from build123d import *
from OCP.BRepFilletAPI import BRepFilletAPI_MakeChamfer

# Parameters (mm, degrees)
BOSS_EXTRUDE2_DEPTH           = 26
SKETCH5_R                     = 11
CUT_EXTRUDE1_DEPTH            = 52.857979135
CSK_FOR_M3_SFHCS1_D           = 3.4
CSK_FOR_M3_SFHCS1_CSINK_D     = 6.72
CSK_FOR_M3_SFHCS1_CSINK_ANGLE = 90
BOSS_EXTRUDE4_DEPTH           = 52
CUT_EXTRUDE2_DEPTH            = 55.481648286
CBORE_FOR_M5_SHCS1_AT_2_COUNT = 2
CBORE_FOR_M5_SHCS1_AT_2_PITCH = 20
SKETCH13_R                    = 5
CUT_EXTRUDE3_DEPTH            = 55.481648286
CUT_EXTRUDE4_DEPTH            = 56.686623169
CHAMFER1_SIZE                 = 1
CHAMFER1_SIZE2                = 0.80190417
CHAMFER2_SIZE                 = 4


with BuildPart() as part:
    # Sketch3 → Boss-Extrude2 (new, symmetric)
    with BuildSketch(Plane(origin=(0, 0, 0), x_dir=(1, 0, 0), z_dir=(0, 1, 0))):
        Polygon((-22.5, -7), (22.5, -7), (22.5, -18), (43.5, -18), (43.5, 0), (-22.5, 0), align=None)
    extrude(amount=BOSS_EXTRUDE2_DEPTH, both=True)

    # Sketch5 → Cut-Extrude1 (cut, through all)
    with BuildSketch(Plane.XY.offset(7)):
        with Locations((-1.35, 0)):
            Circle(SKETCH5_R)
    extrude(amount=-CUT_EXTRUDE1_DEPTH, mode=Mode.SUBTRACT)

    # CSK for M3 SFHCS1 (through all)
    with Locations(Plane.XY.offset(7)):
        with Locations((-16.85, -15.5), (-16.85, 15.5), (14.15, 15.5), (14.15, -15.5)):
            CounterSinkHole(CSK_FOR_M3_SFHCS1_D / 2, CSK_FOR_M3_SFHCS1_CSINK_D / 2, counter_sink_angle=CSK_FOR_M3_SFHCS1_CSINK_ANGLE)

    # Sketch9 → Boss-Extrude4 (add)
    with BuildSketch(Plane(origin=(0, 26, 0), x_dir=(1, 0, 0), z_dir=(0, 1, 0))):
        Polygon((-22.5, 0), (43.5, 20), (43.5, 0), align=None)
    extrude(amount=-BOSS_EXTRUDE4_DEPTH)

    # Sketch10 → Cut-Extrude2 (cut, through all)
    with BuildSketch(Plane.XY):
        Polygon((19.85, -17.089832201), (19.85, 17.089832201), (15.739832201, 21.2), (-18.439832201, 21.2), (-22.55, 17.089832201), (-22.55, -17.089832201), (-18.439832201, -21.2), (15.739832201, -21.2), align=None)
    extrude(amount=-CUT_EXTRUDE2_DEPTH, mode=Mode.SUBTRACT)

    # Sketch12 → CBORE for M5 SHCS1 (revolve, cut)
    with BuildSketch(Plane(origin=(32.5, 9.958578644, 0), x_dir=(0, 1, 0), z_dir=(1, 0, 0))):
        Polygon((0, 0), (0, 18), (2.75, 18), (2.75, 5), (5, 5), (5, 0), align=None)
    cbore_for_m5_shcs1 = revolve(axis=Axis((32.5, 9.958578644, -6.35), (0, 0, 1)), mode=Mode.SUBTRACT)

    # CBORE for M5 SHCS1 at 2: CBORE for M5 SHCS1 ×2
    with Locations(*[(0, -i * CBORE_FOR_M5_SHCS1_AT_2_PITCH, 0) for i in range(1, CBORE_FOR_M5_SHCS1_AT_2_COUNT)]):
        add(cbore_for_m5_shcs1, mode=Mode.SUBTRACT)

    # Sketch13 → Cut-Extrude3 (cut, through all)
    with BuildSketch(Plane.XY):
        with Locations(Location((32.5, -10.041421356, 0), (0, 0, 180))):
            Circle(SKETCH13_R)
        with Locations(Location((32.5, 9.958578644, 0), (0, 0, 180))):
            Circle(SKETCH13_R)
    extrude(amount=-CUT_EXTRUDE3_DEPTH, mode=Mode.SUBTRACT)

    # Sketch14 → Cut-Extrude4 (cut, through all)
    with BuildSketch(Plane.ZY.offset(-22.5)):
        Polygon((7, -26), (18, -20.041421356), (18, -26), align=None)
    cut_extrude4 = extrude(amount=-CUT_EXTRUDE4_DEPTH, mode=Mode.SUBTRACT)

    # Mirror2: Cut-Extrude4 across plane
    add(cut_extrude4.mirror(Plane.ZX), mode=Mode.SUBTRACT)

    # Chamfer1: one chamfer whose edges measure the first distance from different faces: ONE call of the kernel's chamfer builder (chamfer() names one face for all edges)
    chamfer1_edges_1 = [part.edges().sort_by_distance(p)[0] for p in [
        (43.5, -26, -6.5),
        (43.5, -23.020710678, 12.5),
        (43.5, 26, -6.5),
        (43.5, 0, 18),
        (43.5, 23.020710678, 12.5),
    ]]
    chamfer1_edges_2 = [part.edges().sort_by_distance(p)[0] for p in [
        (43.5, 0, -20),
    ]]
    chamfer1_side_2 = [part.faces().sort_by_distance(p)[0] for p in [
        (21.99684701, 0.004301334, -13.483893033),
    ]]
    chamfer1 = BRepFilletAPI_MakeChamfer(part.part.solid().wrapped)
    for e in chamfer1_edges_1:
        chamfer1.Add(CHAMFER1_SIZE, e.wrapped)
    for e in chamfer1_edges_2:
        chamfer1.Add(CHAMFER1_SIZE, CHAMFER1_SIZE2, e.wrapped, chamfer1_side_2[0].wrapped)  # the first distance lies on this face
    add(Compound.cast(chamfer1.Shape()), mode=Mode.REPLACE)

    # Chamfer2
    chamfer2_edges = [part.edges().sort_by_distance(p)[0] for p in [
        (-22.5, 26, 3.5),
        (-22.5, -26, 3.5),
    ]]
    chamfer(chamfer2_edges, length=CHAMFER2_SIZE)


solid = part.part
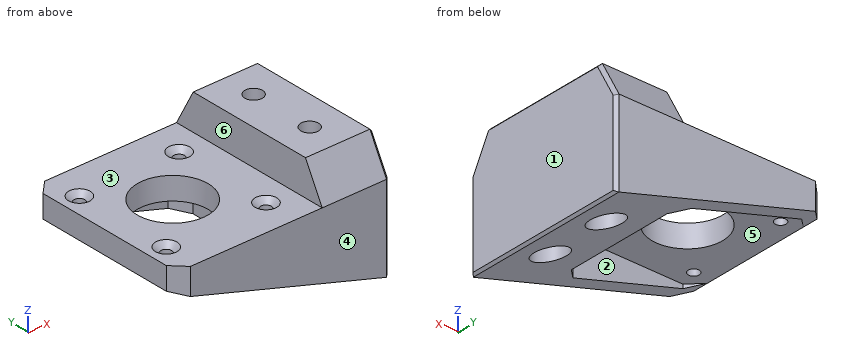
Read the model definition and answer for the solid it produces. Units are mm, in the model's axes. Face numbers are marked on the shaded views. A direction names the side the tool comes from. Coordinates: 2 decimals unless noted, no trailing zeros. Loops run counter-clockwise (first coordinate to the right, second up) from the corner with the lowest first, then second, coordinate; pieces in that order, holes last. Notation, with made-up numbers: (79.5, 8) -> (110.5, 8) arc R30 cw to (110.5, 45) -> close; hole circle Ø1 at (42, -23). An arc over 180 degrees is marked (long way). Write item = value, one per line. Start each with the question number.
1) The part is cut by section C-C, the plane x = -1.35. Determine the outline of the cut face in (y, z), plus the area to 3 significant figures.
2) Given P1, Ø22.5, axis at x = -6, y = 10, coming from the +Z side; P2, Ø1.5, axis at x = 9, y = 10, coming from the -Z side; P3, Ø8, axis at x = 33.5, y = -9, coming from the -Z side, each flat-ended and moving along its own axis, determine where each tip first touches the part or whether it passes through.
3) The part is cut by section A-A, the plane y = 0. Determine the outline of the cut face in (x, z).
4) Find the intervals of material crossed by L1, parallel to Y at x = 32.5, z = -7.5; L2, parallel to X at y = 15.5, z = 3.1; L3, parallel to Y at x = 14.15, z = 3.05, in increasing order. Write a range as from..to.
5) The mould has two halves that part along X. Classify the marked faces 4, 5 and 6: pulls with the +X half, pulls with the -X half, needs draft (parallel to the pull), parting line crosses it, or undercut.
6) For the marked faces 1, 2 and 3, determine the directions among +Z, -Z, +X, -X, +Y, -Y from which every point of the face is accessible in a straight line to the end or side of a thin tool.
7) The part is cut by section D-D, the plane z = -14. Determine the outline of the cut face in (x, y), plus the area to 3 significant figures.
8) The part is cut by section B-B, the plane x = 32.5. Determine the outline of the cut face in (y, z), plus the area to 3 significant figures.
Result:
q1.outline = (-26, -6.41) -> (-21.2, -6.41) -> (-21.2, 0) -> (-11, 0) -> (-11, 7) -> (-26, 7) -> close; (11, 0) -> (21.2, 0) -> (21.2, -6.41) -> (26, -6.41) -> (26, 7) -> (11, 7) -> close
q1.area = 272 mm²
q2.P1 = 7
q2.P2 = 0
q2.P3 = -18.18
q3.outline = (-22.5, 0) -> (-12.35, 0) -> (-12.35, 7) -> (-22.5, 7) -> close; (9.65, 0) -> (19.85, 0) -> (19.85, -12.83) -> (42.54, -19.71) -> (43.5, -19.2) -> (43.5, 17) -> (42.5, 18) -> (22.5, 18) -> (22.5, 7) -> (9.65, 7) -> close
q4.L1 = -26..-15.04, -5.04..4.96, 14.96..26
q4.L2 = -22.5..-18.55, -15.15..12.45, 15.85..43.5
q4.L3 = -26..-17.2, -13.8..13.8, 17.2..26
q5.face_4 = needs draft
q5.face_5 = undercut
q5.face_6 = pulls with the -X half
q6.face_1 = +Z, -Z, +X, +Y, -Y
q6.face_2 = -Z
q6.face_3 = +Z, -X, +Y, -Y
q7.outline = (23.7, -26) -> (42.5, -26) -> (43.5, -25) -> (43.5, 25) -> (42.5, 26) -> (23.7, 26) -> close; hole circle Ø10 at (32.5, -10.04); hole circle Ø10 at (32.5, 9.96)
q7.area = 872 mm²
q8.outline = (-26, -16.67) -> (-15.04, -16.67) -> (-15.04, 5) -> (-12.79, 5) -> (-12.79, 18) -> (-20.04, 18) -> (-26, 7) -> close; (-7.29, 5) -> (-5.04, 5) -> (-5.04, -16.67) -> (4.96, -16.67) -> (4.96, 5) -> (7.21, 5) -> (7.21, 18) -> (-7.29, 18) -> close; (12.71, 5) -> (14.96, 5) -> (14.96, -16.67) -> (26, -16.67) -> (26, 7) -> (20.04, 18) -> (12.71, 18) -> close
q8.area = 1,160 mm²
